Verification items for the finished model (mm, model axes). A direction names the side the tool comes from. Give positions to 0.01 mm unless a question says otherwise; leave off trailing zeros. Write each question's results on one line, items separated by ' | '. Start each with the question number.
```python
from build123d import *

# Parameters (mm, degrees)
SKETCH001_W           = 4.5
SKETCH001_H           = 24
POLARPATTERN001_COUNT = 3
POLARPATTERN_COUNT    = 3


with BuildPart() as body001:
    # Sketch001 → Revolution001 (revolve)
    with BuildSketch(Plane.XZ):
        with Locations((2.25, 12)):
            Rectangle(SKETCH001_W, SKETCH001_H)
    revolution001 = revolve(axis=Axis((0, 0, 0), (0, 0, 1)))

    # PolarPattern001: Revolution001 ×3 about axis
    polarpattern001_axis = Axis((0, 0, 0), (0, 1, 0))
    for i in range(1, POLARPATTERN001_COUNT):
        add(revolution001.rotate(polarpattern001_axis, i * 360 / POLARPATTERN001_COUNT))


with BuildPart() as cut:
    # Sketch → Revolution (revolve)
    with BuildSketch(Plane.XZ):
        Polygon((6.75, 0), (6.75, 10), (6.25, 15.5), (7.75, 15.5), (6.25, 18.098076), (6.25, 19.098076), (7, 19.098076), (6, 23.098076), (0, 23.098076), (0, 0), align=None)
    revolution = revolve(axis=Axis((0, 0, 0), (0, 0, 1)))

    # PolarPattern: Revolution ×3 about axis
    polarpattern_axis = Axis((0, 0, 0), (0, -1, 0))
    for i in range(1, POLARPATTERN_COUNT):
        add(revolution.rotate(polarpattern_axis, i * 360 / POLARPATTERN_COUNT))

    # Cut: cut Body001
    add(body001.part, mode=Mode.SUBTRACT)


solid = cut.part
```
1. Depth check by flat-ended pin: pin 1 Ø5 at (x, y) = (11, -3.5) entering from +Z; pin 2 Ø2 at (x, y) = (12.5, 1.5) entering from -Z; pin 3 Ø2 at (x, y) = (7.5, 6) entering from +Z. Enter the tip coordinate at first touch or a pass-through.
2. Thickness scan on probe 1 along Y at (x, z) = (0, 8); probe 2 along Z at (x, y) = (-10, -1.75); probe 3 along Z at (x, y) = (-10, 2.5). Record the ranges inside material, lowest first.
3. Set-up check for faces 4 (the face through (20.684, 4.472, -10.37)), 5 (the face through (-0.879, 6.693, 6.181)), 6 (the face through (4.292, 1.352, 11.711)): record each of +Z, -Z, +X, -X, +Y, -Y from which the full face is reachable in a straight line by a thin tool's end or side.
4. Release check for a two-part mould opening along X. For faces 1 (the face through (3, 6, 19.098)), 2 (the face through (-12.29, 1.35, -2.14)), 3 (the face through (-19.32, 4.47, -12.73)) record: released by +X, released by -X, zero draft, split by the parting line, or undercut.
5. Section check A-A, the plane y = 0. State how many separate pieces and enclosed holes the cut face has, plus the area to 3 significant figures.
Filled sheet:
1) pin 1: z = 2.25 | pin 2: z = -15.63 | pin 3: z = 1.03
2) probe 1: -6.75 to -4.5, 4.5 to 6.75 | probe 2: -14.28 to -13.68, -12.75 to -10.56, -0.99 to 1.75 | probe 3: -14.1 to -13.68, -12.46 to -10.09, -1.45 to 1.47
3) face 4: -Z, +X, +Y, -Y | face 5: none | face 6: +Z
4) face 1: zero draft | face 2: undercut | face 3: released by -X
5) separate pieces: 3 | enclosed holes: 0 | area: 255 mm2
